Could you check a few things on this model? Use its own coordinates, in mm. Face numbers are marked on the shaded views. A direction names the side the tool comes from. Round coordinates to 2 decimals unless told otherwise and drop trailing zeros. Loops run counter-clockwise (first coordinate to the right, second up) from the corner with the lowest first, then second, coordinate; pieces in that order, holes last. Notation, with made-up numbers: (10.25, -19.75) - (20.25, -19.75) arc R25 ccw to (20.25, 10.25) - close; hole circle Ø6 at (52.25, 73.25). An arc over 180 degrees is marked (long way). Use one line per item in the form item = value.
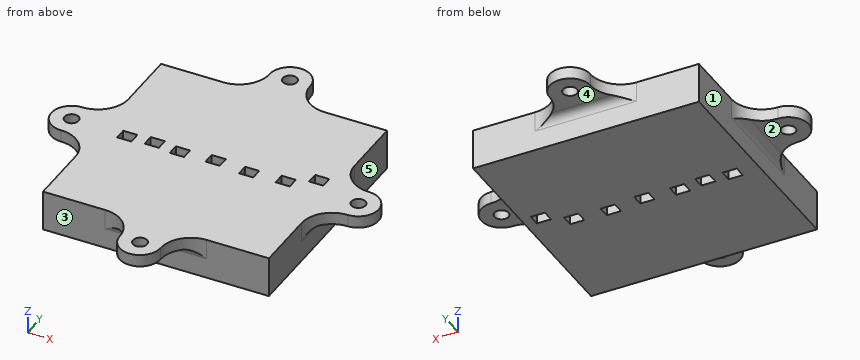
Autodesk Inventor part; units mm, degrees
ref_plane "YZ Plane" through (0, 0, 0) normal (1, 0, 0) x (0, 1, 0)
ref_plane "XZ Plane" through (0, 0, 0) normal (0, 1, 0) x (-1, 0, 0)
ref_plane "XY Plane" through (0, 0, 0) normal (0, 0, 1) x (1, 0, 0)
sketch "Sketch1" plane through (0, 0, 0) normal (0, 0, 1) x (1, 0, 0)
  circle A0 centre (23.5812, 3.9705) radius 1.4165 construction
  circle A1 centre (17.25, 0) radius 1.4165 construction
  circle A2 centre (8.575, 0) radius 1.4165 construction
  circle A3 centre (0, 0) radius 1.4165 construction
  circle A4 centre (-8.4745, 0) radius 1.4165 construction
  circle A5 centre (-15.0058, 0) radius 1.4165 construction
  circle A6 centre (-21.437, 0) radius 1.4165 construction
  line L0 (25.625, 25.625) -> (-25.6245, 25.625) construction
  line L1 (-25.6245, 25.625) -> (-25.6245, -25.625) construction
  line L2 (-25.6245, -25.625) -> (25.625, -25.625) construction
  line L3 (25.625, -25.625) -> (25.625, 25.625) construction
  line L4 (21.8312, 5.4035) -> (25.3312, 5.4035)
  line L5 (25.3312, 5.4035) -> (25.3312, 2.5375)
  line L6 (25.3312, 2.5375) -> (21.8312, 2.5375)
  line L7 (21.8312, 2.5375) -> (21.8312, 5.4035)
  line L8 (21.8312, 5.4035) -> (25.3312, 2.5375) construction
  line L9 (25.3312, 5.4035) -> (21.8312, 2.5375) construction
  line L10 (15.5, 1.75) -> (19, 1.75)
  line L11 (19, 1.75) -> (19, -1.116)
  line L12 (15.5, -1.116) -> (15.5, 1.75)
  line L13 (6.825, 1.116) -> (10.325, 1.116)
  line L14 (10.325, 1.116) -> (10.325, -1.75)
  line L15 (10.325, -1.75) -> (6.825, -1.75)
  line L16 (6.825, -1.75) -> (6.825, 1.116)
  line L17 (-1.75, 1.75) -> (1.75, 1.75)
  line L18 (1.75, 1.75) -> (1.75, -1.116)
  line L19 (-1.75, -1.116) -> (-1.75, 1.75)
  line L20 (-10.2245, 1.116) -> (-6.7245, 1.116)
  line L21 (-6.7245, 1.116) -> (-6.7245, -1.75)
  line L22 (-6.7245, -1.75) -> (-10.2245, -1.75)
  line L23 (-10.2245, -1.75) -> (-10.2245, 1.116)
  line L24 (-16.7558, 1.75) -> (-13.2558, 1.75)
  line L25 (-13.2558, 1.75) -> (-13.2558, -1.116)
  line L26 (-16.7558, -1.116) -> (-16.7558, 1.75)
  line L27 (-23.187, 1.116) -> (-19.687, 1.116)
  line L28 (-19.687, 1.116) -> (-19.687, -1.75)
  line L29 (-19.687, -1.75) -> (-23.187, -1.75)
  line L30 (-23.187, -1.75) -> (-23.187, 1.116)
  line L31 (25.825, 25.825) -> (-25.8245, 25.825)
  line L32 (-25.8245, 25.825) -> (-25.8245, -25.825)
  line L33 (-25.8245, -25.825) -> (25.825, -25.825)
  line L34 (25.825, -25.825) -> (25.825, 25.825)
  line L35 (27.825, 27.825) -> (-27.8245, 27.825)
  line L36 (-27.8245, 27.825) -> (-27.8245, -27.825)
  line L37 (-27.8245, -27.825) -> (27.825, -27.825)
  line L38 (27.825, -27.825) -> (27.825, 27.825)
  line L39 (-16.7558, -1.116) -> (-13.2558, -1.116)
  line L40 (-1.75, -1.116) -> (1.75, -1.116)
  line L41 (15.5, -1.116) -> (19, -1.116)
  point P0 (0, 0)
  point P1 (-16.6189, -1.116)
  dimension "d0" = 3.5
  dimension "d1" = 2.866
  dimension "d4" = 3.5
  dimension "d5" = 2.866
  dimension "d8" = 3.5
  dimension "d9" = 2.866
  dimension "d12" = 3.5
  dimension "d13" = 2.866
  dimension "d14" = 0.2
  dimension "d15" = 2
extrude "Extrusion1" add sketch "Sketch1" along normal blind 10 contours L34 L33 L32 L31 | L38 L37 L36 L35
sketch "Sketch2" plane through (0, 0, 0) normal (0, 0, -1) x (-1, 0, 0)
  line L0 (27.8245, 27.825) -> (27.8245, -27.825)
  line L1 (-27.825, 27.825) -> (27.8245, 27.825)
  line L2 (-27.825, -27.825) -> (-27.825, 27.825)
  line L3 (27.8245, -27.825) -> (-27.825, -27.825)
  line L4 (23.187, -1.75) -> (23.187, 1.116)
  line L5 (19.687, -1.75) -> (23.187, -1.75)
  line L6 (19.687, 1.116) -> (19.687, -1.75)
  line L7 (23.187, 1.116) -> (19.687, 1.116)
  line L8 (10.2245, -1.75) -> (10.2245, 1.116)
  line L9 (6.7245, -1.75) -> (10.2245, -1.75)
  line L10 (6.7245, 1.116) -> (6.7245, -1.75)
  line L11 (10.2245, 1.116) -> (6.7245, 1.116)
  line L12 (-6.825, -1.75) -> (-6.825, 1.116)
  line L13 (-10.325, -1.75) -> (-6.825, -1.75)
  line L14 (-10.325, 1.116) -> (-10.325, -1.75)
  line L15 (-6.825, 1.116) -> (-10.325, 1.116)
  line L16 (-21.8312, 5.4035) -> (-25.3312, 5.4035)
  line L17 (-21.8312, 2.5375) -> (-21.8312, 5.4035)
  line L18 (-25.3312, 2.5375) -> (-21.8312, 2.5375)
  line L19 (-25.3312, 5.4035) -> (-25.3312, 2.5375)
  line L20 (25.8245, -25.825) -> (25.8245, 25.825)
  line L21 (25.8245, 25.825) -> (-25.825, 25.825)
  line L22 (-25.825, 25.825) -> (-25.825, -25.825)
  line L23 (-25.825, -25.825) -> (25.8245, -25.825)
  point P0 (0, 0)
  dimension "d18" = 2
extrude "Extrusion2" [suppressed]
ref_plane "Work Plane1" through (0, 0, 10) normal (0, 0, -1) x (-1, 0, 0)
sketch "Sketch3" plane through (0, 0, 10) normal (0, 0, -1) x (-1, 0, 0)
  circle A0 centre (35.325, 0) radius 1.75
  circle A1 centre (-0.0002, -35.325) radius 1.75
  circle A2 centre (-35.325, 0) radius 1.75
  circle A3 centre (-0.0002, 35.325) radius 1.75
  line L0 (7.4998, 35.325) -> (7.4998, 35.325)
  line L1 (-7.5003, 35.325) -> (-7.5003, 35.325)
  arc A4 (4.9998, 35.325) -> (-5.0002, 35.325) centre (-0.0002, 35.325) ccw
  arc A5 (-35.325, 5) -> (-35.325, -5) centre (-35.325, 0) ccw
  arc A6 (35.325, -5) -> (35.325, 5) centre (35.325, 0) ccw
  arc A7 (-5.0002, -35.325) -> (4.9998, -35.325) centre (-0.0002, -35.325) ccw
  line L2 (27.8245, 27.825) -> (-27.825, 27.825)
  line L3 (27.8245, -27.825) -> (-27.825, -27.825)
  line L4 (-35.325, 5) -> (-35.325, 5)
  line L5 (-5.0002, 35.325) -> (-5.0002, 35.325)
  line L6 (4.9998, 35.325) -> (4.9998, 35.325)
  line L7 (35.325, 5) -> (35.3245, 5)
  line L8 (27.8245, -27.825) -> (27.8245, 27.825)
  line L9 (35.325, -5) -> (35.3245, -5)
  line L10 (4.9998, -35.325) -> (4.9998, -35.325)
  line L11 (-5.0002, -35.325) -> (-5.0002, -35.325)
  line L12 (-35.325, -5) -> (-35.325, -5)
  line L13 (-27.825, -27.825) -> (-27.825, -12.5)
  line L14 (-27.825, 12.5) -> (-27.825, 27.825)
  line L15 (27.8245, -27.825) -> (12.4998, -27.825)
  line L16 (-12.5002, -27.825) -> (-27.825, -27.825)
  line L17 (27.8245, 27.825) -> (27.8245, 12.5)
  line L18 (27.8245, -12.5) -> (27.8245, -27.825)
  line L19 (-27.825, 27.825) -> (-12.5002, 27.825)
  line L20 (12.4998, 27.825) -> (27.8245, 27.825)
  arc A8 (-35.325, 5) -> (-27.825, 12.5) centre (-35.325, 12.5) ccw
  arc A9 (-27.825, -12.5) -> (-35.325, -5) centre (-35.325, -12.5) ccw
  arc A10 (-5.0002, -35.325) -> (-12.5002, -27.825) centre (-12.5002, -35.325) ccw
  arc A11 (12.4998, -27.825) -> (4.9998, -35.325) centre (12.4998, -35.325) ccw
  arc A12 (35.3245, -5) -> (27.8245, -12.5) centre (35.3245, -12.5) ccw
  arc A13 (27.8245, 12.5) -> (35.3245, 5) centre (35.3245, 12.5) ccw
  arc A14 (4.9998, 35.325) -> (12.4998, 27.825) centre (12.4998, 35.325) ccw
  arc A15 (-12.5002, 27.825) -> (-5.0002, 35.325) centre (-12.5002, 35.325) ccw
  line L21 (-27.825, -12.5) -> (-27.825, 12.5)
  line L22 (-25.825, -25.825) -> (-25.825, 25.825)
  point P0 (27.8245, 5)
  point P1 (27.8245, -5)
  point P2 (-5.0002, -35.325)
  point P3 (4.9998, -35.325)
  point P4 (-5.0002, 35.325)
  dimension "d25" = 10
  dimension "d26" = 10
  dimension "d27" = 7.5
extrude "Extrusion3" add sketch "Sketch3" along normal blind 3 contours A14 L2 A15 A4 | A13 A6 A12 L8 | L21 A9 A5 A8 | A11 A7 A10 L3
fillet "Fillet1" radius 2 4 edges at (-27.8245, 0, 7) (0.0002, 27.825, 7) (27.825, 0, 7) (0.0002, -27.825, 7)
sketch "Sketch4" plane through (0, 0, 0) normal (0, 0, -1) x (-1, 0, 0)
  line L0 (27.8245, 27.825) -> (27.8245, -27.825) construction
  line L1 (-27.825, 27.825) -> (27.8245, 27.825) construction
  line L2 (-27.825, -27.825) -> (-27.825, 27.825) construction
  line L3 (27.8245, -27.825) -> (-27.825, -27.825) construction
  line L4 (-21.8312, 5.4035) -> (-25.3312, 5.4035) construction
  line L5 (-21.8312, 2.5375) -> (-21.8312, 5.4035) construction
  line L6 (-25.3312, 2.5375) -> (-21.8312, 2.5375) construction
  line L7 (-25.3312, 5.4035) -> (-25.3312, 2.5375) construction
  line L8 (-15.5, -1.116) -> (-15.5, 1.75) construction
  line L9 (-19, -1.116) -> (-15.5, -1.116) construction
  line L10 (-19, 1.75) -> (-19, -1.116) construction
  line L11 (-15.5, 1.75) -> (-19, 1.75) construction
  line L12 (-6.825, -1.75) -> (-6.825, 1.116) construction
  line L13 (-10.325, -1.75) -> (-6.825, -1.75) construction
  line L14 (-10.325, 1.116) -> (-10.325, -1.75) construction
  line L15 (-6.825, 1.116) -> (-10.325, 1.116) construction
  line L16 (1.75, -1.116) -> (1.75, 1.75) construction
  line L17 (-1.75, -1.116) -> (1.75, -1.116) construction
  line L18 (-1.75, 1.75) -> (-1.75, -1.116) construction
  line L19 (1.75, 1.75) -> (-1.75, 1.75) construction
  line L20 (10.2245, -1.75) -> (10.2245, 1.116) construction
  line L21 (6.7245, -1.75) -> (10.2245, -1.75) construction
  line L22 (6.7245, 1.116) -> (6.7245, -1.75) construction
  line L23 (10.2245, 1.116) -> (6.7245, 1.116) construction
  line L24 (16.7558, -1.116) -> (16.7558, 1.75) construction
  line L25 (13.2558, -1.116) -> (16.7558, -1.116) construction
  line L26 (13.2558, 1.75) -> (13.2558, -1.116) construction
  line L27 (16.7558, 1.75) -> (13.2558, 1.75) construction
  line L28 (23.187, -1.75) -> (23.187, 1.116) construction
  line L29 (19.687, -1.75) -> (23.187, -1.75) construction
  line L30 (19.687, 1.116) -> (19.687, -1.75) construction
  line L31 (23.187, 1.116) -> (19.687, 1.116) construction
  line L32 (26.8245, -26.825) -> (26.8245, 26.825)
  line L33 (26.8245, 26.825) -> (-26.825, 26.825)
  line L34 (-26.825, 26.825) -> (-26.825, -26.825)
  line L35 (-26.825, -26.825) -> (26.8245, -26.825)
  line L36 (24.187, -2.75) -> (24.187, 2.116)
  line L37 (18.687, 2.116) -> (18.687, -2.75)
  line L38 (17.7558, -2.116) -> (17.7558, 2.75)
  line L39 (12.2558, 2.75) -> (12.2558, -2.116)
  line L40 (11.2245, -2.75) -> (11.2245, 2.116)
  line L41 (5.7245, 2.116) -> (5.7245, -2.75)
  line L42 (2.75, -2.116) -> (2.75, 2.75)
  line L43 (-2.75, 2.75) -> (-2.75, -2.116)
  line L44 (-5.825, -2.75) -> (-5.825, 2.116)
  line L45 (-11.325, 2.116) -> (-11.325, -2.75)
  line L46 (-14.5, 2.75) -> (-14.5, -2.116)
  line L47 (-20, -2.116) -> (-20, 2.75)
  line L48 (-20.8312, 1.5375) -> (-20.8312, 6.4035)
  line L49 (-26.3312, 6.4035) -> (-26.3312, 1.5375)
  line L50 (-23.5812, 26.825) -> (-23.5812, -26.825) construction
  line L51 (-17.25, 26.825) -> (-17.25, -26.825) construction
  line L52 (-0.0002, 26.825) -> (-0.0003, -26.825) construction
  line L53 (8.4745, -26.825) -> (8.4745, 26.825) construction
  line L54 (15.0058, 26.825) -> (15.0057, -26.825) construction
  line L55 (21.437, -26.825) -> (21.437, 26.825) construction
  line L56 (-22.5812, 26.825) -> (-22.5812, 6.4035)
  line L57 (-22.5812, 1.5375) -> (-22.5812, -26.825)
  line L58 (-24.5812, 26.825) -> (-24.5812, 6.4035)
  line L59 (-24.5812, 1.5375) -> (-24.5812, -26.825)
  line L60 (-26.3312, 1.5375) -> (-24.5812, 1.5375)
  line L61 (-22.5812, 1.5375) -> (-20.8312, 1.5375)
  line L62 (-20.8312, 6.4035) -> (-22.5812, 6.4035)
  line L63 (-24.5812, 6.4035) -> (-26.3312, 6.4035)
  line L64 (-20, 2.75) -> (-18.25, 2.75)
  line L65 (-16.25, 2.75) -> (-14.5, 2.75)
  line L66 (-16.25, 26.825) -> (-16.25, 2.75)
  line L67 (-16.25, -2.116) -> (-16.25, -26.825)
  line L68 (-18.25, 26.825) -> (-18.25, 2.75)
  line L69 (-18.25, -2.116) -> (-18.25, -26.825)
  line L70 (-14.5, -2.116) -> (-16.25, -2.116)
  line L71 (-18.25, -2.116) -> (-20, -2.116)
  line L72 (-11.325, -2.75) -> (-9.575, -2.75)
  line L73 (-7.575, -2.75) -> (-5.825, -2.75)
  line L74 (-5.825, 2.116) -> (-7.575, 2.116)
  line L75 (-9.575, 2.116) -> (-11.325, 2.116)
  line L76 (2.75, 2.75) -> (0.9998, 2.75)
  line L77 (-1.0002, 2.75) -> (-2.75, 2.75)
  line L78 (0.9998, 26.825) -> (0.9998, 2.75)
  line L79 (0.9998, -2.116) -> (0.9998, -26.825)
  line L80 (-2.75, -2.116) -> (-1.0002, -2.116)
  line L81 (0.9998, -2.116) -> (2.75, -2.116)
  line L82 (-1.0002, 26.825) -> (-1.0002, 2.75)
  line L83 (-1.0002, -2.116) -> (-1.0002, -26.825)
  line L84 (11.2245, 2.116) -> (9.4745, 2.116)
  line L85 (7.4745, 2.116) -> (5.7245, 2.116)
  line L86 (9.4745, -26.825) -> (9.4745, -2.75)
  line L87 (9.4745, 2.116) -> (9.4745, 26.825)
  line L88 (5.7245, -2.75) -> (7.4745, -2.75)
  line L89 (9.4745, -2.75) -> (11.2245, -2.75)
  line L90 (7.4745, -26.825) -> (7.4745, -2.75)
  line L91 (7.4745, 2.116) -> (7.4745, 26.825)
  line L92 (14.0058, 26.825) -> (14.0058, 2.75)
  line L93 (16.0058, 26.825) -> (16.0058, 2.75)
  line L94 (16.0058, -2.116) -> (16.0057, -26.825)
  line L95 (14.0058, -2.116) -> (14.0057, -26.825)
  line L96 (20.437, 2.116) -> (20.437, 26.825)
  line L97 (22.437, -26.825) -> (22.437, -2.75)
  line L98 (22.437, 2.116) -> (22.437, 26.825)
  line L99 (24.187, 2.116) -> (22.437, 2.116)
  line L100 (20.437, 2.116) -> (18.687, 2.116)
  line L101 (17.7558, 2.75) -> (16.0058, 2.75)
  line L102 (14.0058, 2.75) -> (12.2558, 2.75)
  line L103 (12.2558, -2.116) -> (14.0058, -2.116)
  line L104 (16.0058, -2.116) -> (17.7558, -2.116)
  line L105 (20.437, -26.825) -> (20.437, -2.75)
  line L106 (18.687, -2.75) -> (20.437, -2.75)
  line L107 (22.437, -2.75) -> (24.187, -2.75)
  line L108 (-8.575, 26.825) -> (-8.575, -26.825) construction
  line L109 (-7.575, 26.825) -> (-7.575, 2.116)
  line L110 (-7.575, -2.75) -> (-7.575, -26.825)
  line L111 (-9.575, 26.825) -> (-9.575, 2.116)
  line L112 (-9.575, -2.75) -> (-9.575, -26.825)
  point P0 (0, 0)
  dimension "d4" = 3.5
  dimension "d5" = 2.866
extrude "Extrusion4" [suppressed]
properties part number "frame"
1. If we section it at B-B, the plane x = -14.5: Write out the boundary of the cut face in (y, z) (3 decimals), plus the area to 3 significant figures.
Solution:
outline = (-27.825, 0) - (-1.116, 0) - (-1.116, 10) - (-27.825, 10) - close; (1.75, 0) - (27.825, 0) - (27.825, 10) - (1.75, 10) - close
area = 528 mm^2
2. On a 3-axis mill with a long thin cutter (end or side, diameter ignored), from which of +Z, -Z, +X, -X, +Y, -Y can I reach the whole of each face in a straight line? I mean the marked faces 1, 2, 3, 4 and 5. Say none if no direction works.
Solution:
face_1 = -Z, -X
face_2 = -Z, -X, +Y, -Y
face_3 = -Z, -Y
face_4 = -Z, +X, -X, +Y
face_5 = -Z, +X
3. For P1, Ø1.8, axis at x = -14.5, z = 6, coming from the +Y side (3 decimals); P2, Ø1.8, axis at x = -15.5, z = 3.5, coming from the -Y side (3 decimals); P3, Ø4, axis at x = 0, y = 35.33, coming from the -Z side; P4, Ø3, axis at x = 35.325, y = 0, coming from the -Z side, each with a flat end and sliding along its axis, tell me the tip position at first contact or that it passes through.
Solution:
P1 = 27.825
P2 = -27.825
P3 = 7
P4 = through
4. If we section it at D-D, the plane x = -3: Write out the boundary of the cut face in (y, z) (3 decimals), plus the area to 3 significant figures.
Solution:
outline = (-39.325, 7) - (-29.825, 7) arc R2 cw to (-27.825, 5) - (-27.825, 0) - (27.825, 0) - (27.825, 5) arc R2 cw to (29.825, 7) - (39.325, 7) - (39.325, 10) - (-39.325, 10) - close
area = 627 mm^2
5. Please list where these lines run through material, in increasing order: line 1 along X through (y, z) = (35.5, 7.25); line 2 along Y through (x, z) = (-20, 9.75) (3 decimals); line 3 along X through (y, z) = (-23.5, 6.75) (1 decimal).
Solution:
line_1 = -5 to -1.74, 1.74 to 5
line_2 = -27.825 to -1.75, 1.116 to 27.825
line_3 = -27.8 to 27.8
6. If we section it at A-A, the plane z = 1: Count the separate pieces of the cut face and the enclosed holes in it, plus the area to 3 significant figures.
Solution:
separate_pieces = 1
enclosed_holes = 7
area = 3,030 mm^2
